Part model, mm, in its own coordinate system. Face numbers are marked on the shaded views. A direction names the side the tool comes from. Round coordinates to 2 decimals unless told otherwise and drop trailing zeros. Write each loop counter-clockwise with the first axis right and the second up, starting at its lowest first coordinate (ties: lowest second). Pieces come first, ordered by that corner, then holes. Notation, with made-up numbers: (-37, 20.25) -> (18, 20.25) arc R22 ccw to (18, 50.25) -> close; hole circle Ø2 at (12.25, 17). An arc over 180 degrees is marked (long way). Use CSV: the item, a comma, the result in double quotes. Start each with the question number.
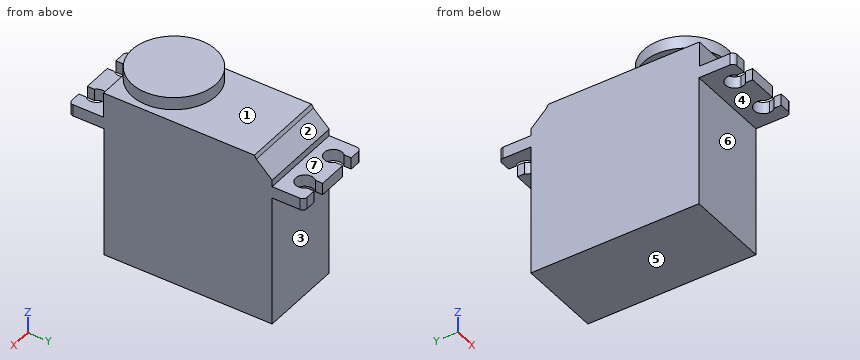
```python
from build123d import *

# Parameters (mm, degrees)
SKETCH1_R           = 2.71138536
BOSS_EXTRUDE2_DEPTH = 2.8
FILLET1_R           = 1
BOSS_EXTRUDE4_REACH = 71.688
SKETCH5_W           = 31.2
SKETCH5_H           = 40
CUT_EXTRUDE1_DEPTH  = 143.310868606
SKETCH7_W           = 29.686403428
SKETCH7_H           = 9.387658688
SKETCH7_W_2         = 27.535306267
SKETCH7_H_2         = 10.174748845
CUT_EXTRUDE2_DEPTH  = 143.310868606
SKETCH9_R           = 3.527564699
BOSS_EXTRUDE5_DEPTH = 4.45
SKETCH8_W           = 7.436989159
SKETCH8_H           = 16.512703909
CUT_EXTRUDE4_DEPTH  = 77.302474202
SKETCH11_R          = 5
BOSS_EXTRUDE6_DEPTH = 1.45
SKETCH12_R          = 10
BOSS_EXTRUDE7_DEPTH = 3


with BuildPart() as part:
    # Sketch1 → Boss-Extrude2 (new body)
    with BuildSketch(Plane.XY):
        with BuildLine():
            Line((101.027913119, 66.698032725), (101.027913119, 10.698032725))
            Line((101.027913119, 10.698032725), (104.53416083, 10.698032725))
            Line((104.53416083, 10.698032725), (104.53416083, 12.400036101))
            ThreePointArc((104.53416083, 12.400036101), (105.187004527, 15.928048429), (108.179096386, 13.948032725))
            ThreePointArc((108.179096386, 13.948032725), (108.007928823, 13.107124133), (107.521665407, 12.400036101))
            Line((107.521665407, 12.400036101), (107.521665407, 10.698032725))
            Line((107.521665407, 10.698032725), (114.53416083, 10.698032725))
            Line((114.53416083, 10.698032725), (114.53416083, 12.400036101))
            ThreePointArc((114.53416083, 12.400036101), (115.187004527, 15.928048429), (118.179096386, 13.948032725))
            ThreePointArc((118.179096386, 13.948032725), (118.007928823, 13.107124133), (117.521665407, 12.400036101))
            Line((117.521665407, 12.400036101), (117.521665407, 10.698032725))
            Line((117.521665407, 10.698032725), (121.027913119, 10.698032725))
            Line((121.027913119, 10.698032725), (121.027913119, 66.698032725))
            Line((121.027913119, 66.698032725), (117.521665407, 66.698032725))
            Line((117.521665407, 66.698032725), (117.521665407, 64.996029349))
            ThreePointArc((117.521665407, 64.996029349), (118.007928823, 64.288941317), (118.179096386, 63.448032725))
            ThreePointArc((118.179096386, 63.448032725), (115.187004527, 61.468017021), (114.53416083, 64.996029349))
            Line((114.53416083, 64.996029349), (114.53416083, 66.698032725))
            Line((114.53416083, 66.698032725), (107.521665407, 66.698032725))
            Line((107.521665407, 66.698032725), (107.521665407, 64.996029349))
            ThreePointArc((107.521665407, 64.996029349), (108.007928823, 64.288941317), (108.179096386, 63.448032725))
            ThreePointArc((108.179096386, 63.448032725), (105.187004527, 61.468017021), (104.53416083, 64.996029349))
            Line((104.53416083, 64.996029349), (104.53416083, 66.698032725))
            Line((104.53416083, 66.698032725), (101.027913119, 66.698032725))
        make_face()
        with Locations((111.027913119, 28.948032725)):
            Circle(SKETCH1_R, mode=Mode.SUBTRACT)
    extrude(amount=BOSS_EXTRUDE2_DEPTH)

    # Fillet1
    fillet1_edges = [part.edges().sort_by_distance(p)[0] for p in [
        (101.027913119, 10.698032725, 1.4),
        (101.027913119, 66.698032725, 1.4),
        (121.027913119, 66.698032725, 1.4),
        (121.027913119, 10.698032725, 1.4),
    ]]
    fillet(fillet1_edges, radius=FILLET1_R)

    # Boss-Extrude4: up to this face of the body (flat: up to its plane)
    boss_extrude4_end = Plane(part.part.faces().sort_by_distance((121.027913119, 38.698032725, 1.4))[0])
    # Sketch5 → Boss-Extrude4 (add, up to the picked face)
    with BuildSketch(Plane.ZY.offset(-101.027913119), mode=Mode.PRIVATE) as boss_extrude4_sk1:
        Polygon((4.36856715, 64.103331084), (2.8, 64.103331084), (2.8, 13.685897531), (3.764993714, 13.685897531), (3.764993714, 18.958103522), (8.8, 18.958103522), (8.8, 22.695834212), (9.718562106, 23.589991727), (9.718562106, 25.946850167), (13.25, 25.946850167), (13.25, 32.391247199), (9.718562106, 32.391247199), (9.718562106, 35.074245433), (8.8, 35.635588942), (8.8, 54.857740136), (8.029983718, 55.328305642), (4.432571629, 59.081605588), (4.36856715, 59.081605588), align=None)
    boss_extrude4_tool1 = split(extrude(boss_extrude4_sk1.sketch, amount=-BOSS_EXTRUDE4_REACH, mode=Mode.PRIVATE), bisect_by=boss_extrude4_end, keep=Keep.BOTH, mode=Mode.PRIVATE)
    # Sketch5 → Boss-Extrude4 (add, up to the picked face)
    with BuildSketch(Plane.ZY.offset(-101.027913119), mode=Mode.PRIVATE) as boss_extrude4_sk2:
        with Locations((-15.6, 39.081605588)):
            Rectangle(SKETCH5_W, SKETCH5_H)
    boss_extrude4_tool2 = split(extrude(boss_extrude4_sk2.sketch, amount=-BOSS_EXTRUDE4_REACH, mode=Mode.PRIVATE), bisect_by=boss_extrude4_end, keep=Keep.BOTH, mode=Mode.PRIVATE)
    add(boss_extrude4_tool1.solids().sort_by(Axis((101.027913, 37.386075, 6.241915), (1, 0, 0)))[0])
    add(boss_extrude4_tool2.solids().sort_by(Axis((101.027913, 39.081606, -15.6), (1, 0, 0)))[0])

    # Sketch6 → Cut-Extrude1 (cut, through all)
    with BuildSketch(Plane(origin=(0, 0, 2.8), x_dir=(-1, 0, 0), z_dir=(0, 0, -1))):
        with BuildLine():
            Line((-113.978968632, 64.103331084), (-118.076857605, 64.103331084))
            ThreePointArc((-118.076857605, 64.103331084), (-116.027913119, 61.296849458), (-113.978968632, 64.103331084))
        make_face()
        with BuildLine():
            Line((-103.978968632, 64.103331084), (-108.076857605, 64.103331084))
            ThreePointArc((-108.076857605, 64.103331084), (-106.027913119, 61.296849458), (-103.978968632, 64.103331084))
        make_face()
        with BuildLine():
            Line((-118.163065242, 13.685897531), (-113.892760996, 13.685897531))
            ThreePointArc((-113.892760996, 13.685897531), (-116.027913119, 16.099215992), (-118.163065242, 13.685897531))
        make_face()
        with BuildLine():
            Line((-108.163065242, 13.685897531), (-103.892760996, 13.685897531))
            ThreePointArc((-103.892760996, 13.685897531), (-106.027913119, 16.099215992), (-108.163065242, 13.685897531))
        make_face()
    extrude(amount=-CUT_EXTRUDE1_DEPTH, mode=Mode.SUBTRACT)

    # Sketch7 → Cut-Extrude2 (cut, through all)
    with BuildSketch(Plane.XY.offset(2.8)):
        with Locations((110.258958877, 63.775434932)):
            Rectangle(SKETCH7_W, SKETCH7_H)
        with Locations((111.334507458, 13.8707291)):
            Rectangle(SKETCH7_W_2, SKETCH7_H_2)
    extrude(amount=CUT_EXTRUDE2_DEPTH, mode=Mode.SUBTRACT)

    # Sketch8 → Cut-Extrude4 (cut, through all)
    with BuildSketch(Plane.ZY.offset(-101.027913119)):
        with Locations((12.51849458, 29.114960016)):
            Rectangle(SKETCH8_W, SKETCH8_H)
    extrude(amount=-CUT_EXTRUDE4_DEPTH, mode=Mode.SUBTRACT)



with BuildPart() as body_2:
    # Sketch9 → Boss-Extrude5 (new, through all)
    with BuildSketch(Plane.XY.offset(8.8)):
        with Locations((111.027913119, 28.948032725)):
            Circle(SKETCH9_R)
    extrude(amount=BOSS_EXTRUDE5_DEPTH)


with BuildPart() as part_1:
    add(part.part)

    add(body_2.part)  # Boss-Extrude6 merges body 2
    # Sketch11 → Boss-Extrude6 (add)
    with BuildSketch(Plane.XY.offset(8.8)):
        with Locations((111.027913119, 28.948032725)):
            Circle(SKETCH11_R)
    extrude(amount=BOSS_EXTRUDE6_DEPTH)

    # Sketch12 → Boss-Extrude7 (add)
    with BuildSketch(Plane.XY.offset(10.25)):
        with Locations((111.027913119, 28.948032725)):
            Circle(SKETCH12_R)
    extrude(amount=BOSS_EXTRUDE7_DEPTH)


solid = part_1.part
```
1. Band-saw the part on B-B (z = 1.5). List the corners of the cut face in (x, y), then the cut area to 3 significant figures.
2. Which spindle directions (+Z, -Z, +X, -X, +Y, -Y) get a long thin tool onto all of the face, cutting with end or side? Do the marked faces 5, 6 and 7. Say none if no direction does.
3. Band-saw the part on A-A (x = 109). List the corners of the cut face in (y, z), then the cut area to 3 significant figures.
4. Band-saw the part on D-D (x = 113). List the corners of the cut face in (y, z), then the cut area to 3 significant figures.
5. Drill centre lines: line 1 along X through (y, z) = (15.5, 1.5); line 2 along X through (y, z) = (63.5, 1); line 3 along Z through (x, y) = (104.5, 32). Where is each one in solid material? Low to high. Write a range as [from, to].
6. Pull direction Z, two halves, no side cores. Call the marked faces 1, 2, 3 and 4: released by +Z, released by -Z, zero draft, split by the parting line, or undercut.
7. Flat gauge pins, fed straight in: pin 1 (10 mm diameter, centred on x = 113.5, z = -13, fed in from +Y); pin 2 (1.3 mm diameter, centred on x = 106, z = 3, fed in from +Y); pin 3 (4 mm diameter, centred on x = 115.5, y = 64.5, fed in from +Z). Where does each tip first touch, or does it go through?
8. Band-saw the part on C-C (y = 53). List the corners of the cut face in (x, z).
Answers below:
1,outline,"(101.03, 11.7) arc R1 ccw to (102.03, 10.7) -> (104.53, 10.7) -> (104.53, 12.4) arc R2.15 cw (long way) to (107.52, 12.4) -> (107.52, 10.7) -> (114.53, 10.7) -> (114.53, 12.4) arc R2.15 cw (long way) to (117.52, 12.4) -> (117.52, 10.7) -> (120.03, 10.7) arc R1 ccw to (121.03, 11.7) -> (121.03, 65.7) arc R1 ccw to (120.03, 66.7) -> (117.52, 66.7) -> (117.52, 65) arc R2.15 cw (long way) to (114.53, 65) -> (114.53, 66.7) -> (107.52, 66.7) -> (107.52, 65) arc R2.15 cw (long way) to (104.53, 65) -> (104.53, 66.7) -> (102.03, 66.7) arc R1 ccw to (101.03, 65.7) -> close; hole circle Ø5.42 at (111.03, 28.95)"
1,area,"1,020 mm^2"
2,face 5,"-Z, +X, -X, +Y, -Y"
2,face 6,"-Z, +X, -X, -Y"
2,face 7,"+Z, +X, -X, +Y"
3,outline,"(10.7, 0) -> (19.08, 0) -> (19.08, -31.2) -> (59.08, -31.2) -> (59.08, 0) -> (66.7, 0) -> (66.7, 2.8) -> (59.08, 2.8) -> (59.08, 4.43) -> (55.33, 8.03) -> (54.86, 8.8) -> (33.52, 8.8) -> (33.52, 10.25) -> (38.74, 10.25) -> (38.74, 13.25) -> (19.16, 13.25) -> (19.16, 10.25) -> (24.38, 10.25) -> (24.38, 8.8) -> (18.96, 8.8) -> (18.96, 2.8) -> (10.7, 2.8) -> close; hole (27.15, 0) -> (30.75, 0) -> (30.75, 2.8) -> (27.15, 2.8) -> close"
3,area,"1,700 mm^2"
4,outline,"(10.7, 0) -> (19.08, 0) -> (19.08, -31.2) -> (59.08, -31.2) -> (59.08, 0) -> (66.7, 0) -> (66.7, 2.8) -> (59.08, 2.8) -> (59.08, 4.43) -> (55.33, 8.03) -> (54.86, 8.8) -> (33.54, 8.8) -> (33.54, 10.25) -> (38.75, 10.25) -> (38.75, 13.25) -> (19.14, 13.25) -> (19.14, 10.25) -> (24.35, 10.25) -> (24.35, 8.8) -> (18.96, 8.8) -> (18.96, 2.8) -> (10.7, 2.8) -> close; hole (27.09, 0) -> (30.81, 0) -> (30.81, 2.8) -> (27.09, 2.8) -> close"
4,area,"1,700 mm^2"
5,line 1,"x = [101.03, 104.54], [107.52, 114.54], [117.52, 121.03]"
5,line 2,"x = [101.03, 103.88], [108.18, 113.88], [118.18, 121.03]"
5,line 3,"z = [-31.2, 8.8], [10.25, 13.25]"
6,face 1,"undercut"
6,face 2,"released by +Z"
6,face 3,"zero draft"
6,face 4,"released by -Z"
7,pin 1,"stops at y = 59.08"
7,pin 2,"stops at y = 61.4"
7,pin 3,"stops at z = 2.8"
8,outline,"(101.03, -31.2) -> (121.03, -31.2) -> (121.03, 8.8) -> (101.03, 8.8) -> close"
